Verification items for the finished model (mm, model axes). A direction names the side the tool comes from. Coordinates: 2 decimals unless noted, no trailing zeros. Loops run counter-clockwise (first coordinate to the right, second up) from the corner with the lowest first, then second, coordinate; pieces in that order, holes last. Notation, with made-up numbers: (-7.75, 86) - (39.25, 86) arc R24 ccw to (39.25, 98) - close; hole circle Ø8 at (27.25, -39.5). An arc over 180 degrees is marked (long way). One line per item, written item: value. Start each with the question number.
(1) Gauge pin test, flat ends, axial feed: P1, Ø1, axis at x = -8, z = 7.5, coming from the +Y side; P2, Ø20, axis at x = -2, z = 3.5, coming from the -Y side; P3, Ø12.5, axis at x = 0, z = 0, coming from the -Y side. Record the tip position at first contact, or that the pin passes through.
(2) Set-up check for faces 4 (the face through (2, 10, 6)), 5 (the face through (-13.5, -6, 0)), 6 (the face through (7, -13, -12)): record each of +Z, -Z, +X, -X, +Y, -Y from which the full face is reachable in a straight line by a thin tool's end or side.
(3) Section check A-A (y = -2.5). Record the boundary of the cut face in (x, z).
(4) Section check B-B (y = 5). Record the boundary of the cut face in (x, z).
(5) Thickness scan on probe 1 along Z at (x, y) = (-0.5, -17); probe 2 along X at (y, z) = (18, 0); probe 3 along X at (y, z) = (-20.75, 0). Record the ranges inside material, lowest first. Write a range as [from, to].
(6) Draft check along X on faces 1 (the face through (-7.91, -18.423, 10.316)), 2 (the face through (-6.656, -5.605, -11.746)), 3 (the face through (7, 25, -2)). Enter one of: +X half, -X half, draft (parallel to the pull), parting line (faces both ways), or undercut.
```python
from build123d import *

# Parameters (mm, degrees)
SKETCH2_R           = 9
BOSS_EXTRUDE2_DEPTH = 15


with BuildPart() as part:
    # Sketch1 → Revolve1 (revolve)
    with BuildSketch(Plane(origin=(0, 0, 0), x_dir=(0, 0, -1), z_dir=(1, 0, 0))):
        with BuildLine():
            Line((13, -24), (13, -13))
            Line((13, -13), (18.02920611, -13))
            ThreePointArc((18.02920611, -13), (19.317404153, -13.470115755), (20, -14.659454198))
            Line((20, -14.659454198), (18, -14.659454198))
            Line((18, -14.659454198), (18, -25))
            Line((18, -25), (14.151715331, -25))
            Line((14.151715331, -25), (13, -24))
        make_face()
        Polygon((10, 25), (7, 25), (7, 16.3), (6, 15.3), (6, 10), (7, 10), (7, 2), (12, 2), (12, 13), (10, 14), align=None)
    revolve(axis=Axis((0, 25, 0), (0, -1, 0)))

    # Sketch2 → Boss-Extrude2 (add)
    with BuildSketch(Plane(origin=(0, -13, 0), x_dir=(1, 0, 0), z_dir=(0, 1, 0))):
        Polygon((0, 15.588457268), (-13.5, 7.794228634), (-13.5, -7.794228634), (0, -15.588457268), (13.5, -7.794228634), (13.5, 7.794228634), align=None)
        Circle(SKETCH2_R, mode=Mode.SUBTRACT)
    extrude(amount=BOSS_EXTRUDE2_DEPTH)


solid = part.part
```
Responses:
1. P1: stops at y = 13.77
1. P2: stops at y = -24.9
1. P3: stops at y = 10
2. face 4: -Y
2. face 5: +Z, -Z, -X, +Y
2. face 6: +Y
3. outline: (-13.5, -7.79) - (0, -15.59) - (13.5, -7.79) - (13.5, 7.79) - (0, 15.59) - (-13.5, 7.79) - close; hole circle Ø18 at (0, 0)
4. outline: circle Ø24 at (0, 0); hole circle Ø14 at (0, 0)
5. probe 1: z = [-17.99, -12.99], [12.99, 17.99]
5. probe 2: x = [-10, -7], [7, 10]
5. probe 3: x = [-18, -13], [13, 18]
6. face 1: undercut
6. face 2: -X half
6. face 3: draft
